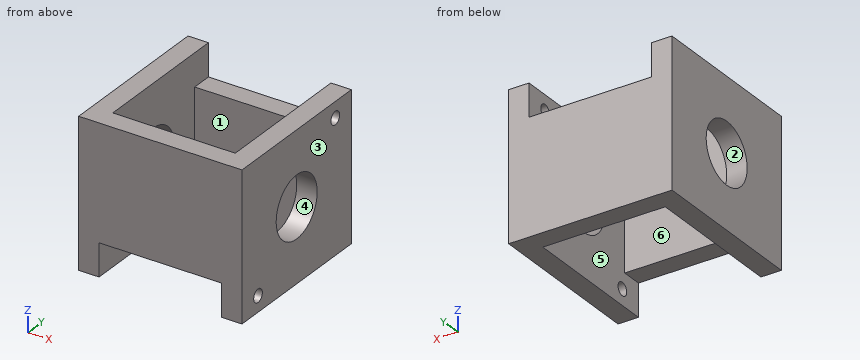
```python
from build123d import *

# Parameters (mm, degrees)
SKETCH1_W                      = 50.8
SKETCH1_H                      = 50.8
SKETCH1_W_2                    = 38.1
SKETCH1_H_2                    = 38.1
EXTRUDE_THIN1_DEPTH            = 45.72
SKETCH2_R                      = 2.0193
CUT_EXTRUDE2_DEPTH             = 1
CUT_EXTRUDE2_DEPTH_BACK        = 6.35
SKETCH4_R                      = 9.525
CUT_EXTRUDE3_DEPTH             = 1
CUT_EXTRUDE3_DEPTH_BACK        = 51.8
CUT_EXTRUDE4_REACH             = 52.8
SKETCH5_W                      = 38.1
SKETCH5_H                      = 10.16
CUT_EXTRUDE4_DIRECTION_2_DEPTH = 1
CUT_EXTRUDE5_START             = -25.4
SKETCH5_3_W                    = 38.1
SKETCH5_3_H                    = 10.16
CUT_EXTRUDE5_DEPTH             = 25.4


with BuildPart() as part:
    # Sketch1 → Extrude-Thin1 (new body)
    with BuildSketch(Plane.XY):
        Rectangle(SKETCH1_W, SKETCH1_H)
        Rectangle(SKETCH1_W_2, SKETCH1_H_2, mode=Mode.SUBTRACT)
    extrude(amount=EXTRUDE_THIN1_DEPTH)

    # Sketch2 → Cut-Extrude2 (cut, two sides)
    with BuildSketch(Plane(origin=(25.4, 0, 0), x_dir=(0, 0, -1), z_dir=(1, 0, 0))) as cut_extrude2_sk:
        with Locations((-40.820512212, 17.96051224)):
            Circle(SKETCH2_R)
        with Locations((-4.899487788, -17.96051224)):
            Circle(SKETCH2_R)
    extrude(amount=CUT_EXTRUDE2_DEPTH, mode=Mode.SUBTRACT)
    extrude(cut_extrude2_sk.sketch, amount=-CUT_EXTRUDE2_DEPTH_BACK, mode=Mode.SUBTRACT)

    # Sketch4 → Cut-Extrude3 (cut, two sides)
    with BuildSketch(Plane(origin=(25.4, 0, 0), x_dir=(0, 0, -1), z_dir=(1, 0, 0))) as cut_extrude3_sk:
        with Locations((-22.86, 0)):
            Circle(SKETCH4_R)
    extrude(amount=CUT_EXTRUDE3_DEPTH, mode=Mode.SUBTRACT)
    extrude(cut_extrude3_sk.sketch, amount=-CUT_EXTRUDE3_DEPTH_BACK, mode=Mode.SUBTRACT)

    # Sketch5 → Cut-Extrude4 (cut, up to next)
    with BuildSketch(Plane.XZ.offset(25.4), mode=Mode.PRIVATE) as cut_extrude4_sk1:
        with Locations((0, 5.08)):
            Rectangle(SKETCH5_W, SKETCH5_H)
    cut_extrude4_tool1 = extrude(cut_extrude4_sk1.sketch, amount=-CUT_EXTRUDE4_REACH, mode=Mode.PRIVATE) & part.part
    add(cut_extrude4_tool1.solids().sort_by_distance((0, -25.4, 5.08))[0], mode=Mode.SUBTRACT)

    # Sketch5 → Cut-Extrude4 direction 2 (cut)
    with BuildSketch(Plane.XZ.offset(25.4)):
        with Locations((0, 5.08)):
            Rectangle(SKETCH5_W, SKETCH5_H)
    extrude(amount=CUT_EXTRUDE4_DIRECTION_2_DEPTH, mode=Mode.SUBTRACT)

    # Sketch5<3> → Cut-Extrude5 (cut)
    with BuildSketch(Plane.XZ.offset(25.4).offset(CUT_EXTRUDE5_START)):
        with Locations((0, 40.64)):
            Rectangle(SKETCH5_3_W, SKETCH5_3_H)
    extrude(amount=-CUT_EXTRUDE5_DEPTH, mode=Mode.SUBTRACT)


solid = part.part
```
Geometry check sheet. Reference: the model listing, model coordinates, mm. Face numbers are marked on the shaded views. A direction names the side the tool comes from. Round coordinates to 2 decimals unless told otherwise and drop trailing zeros. Write each loop counter-clockwise with the first axis right and the second up, starting at its lowest first coordinate (ties: lowest second). Pieces come first, ordered by that corner, then holes. Notation, with made-up numbers: (66, 52.25) -> (115, 52.25) arc R8 ccw to (115, 60.25) -> close; hole circle Ø4 at (26.25, 5). An arc over 180 degrees is marked (long way). Put each result on its own line as item: value.
1) Cross-section at A-A, the plane y = 13. Enter the section's corners in (x, z).
Recorded:
outline: (-25.4, 0) -> (-19.05, 0) -> (-19.05, 45.72) -> (-25.4, 45.72) -> close; (19.05, 0) -> (25.4, 0) -> (25.4, 45.72) -> (19.05, 45.72) -> close
2) Cross-section at B-B, the plane y = 0. Enter the section's corners in (x, z) (3 decimals), plus the area to 3 significant figures.
Recorded:
outline: (-25.4, 0) -> (-19.05, 0) -> (-19.05, 13.335) -> (-25.4, 13.335) -> close; (-25.4, 32.385) -> (-19.05, 32.385) -> (-19.05, 45.72) -> (-25.4, 45.72) -> close; (19.05, 0) -> (25.4, 0) -> (25.4, 13.335) -> (19.05, 13.335) -> close; (19.05, 32.385) -> (25.4, 32.385) -> (25.4, 45.72) -> (19.05, 45.72) -> close
area: 339 mm2
3) Depth check by flat-ended pin: P1, Ø4, axis at x = 3.5, z = 6, coming from the -Y side; P2, Ø7, axis at x = 7, y = 23, coming from the +Z side; P3, Ø3, axis at x = 3, y = -23, coming from the -Z side. Enter the tip coordinate at first touch or a pass-through.
Recorded:
P1: stops at y = 19.05
P2: stops at z = 35.56
P3: stops at z = 10.16
4) Cross-section at C-C, the plane z = 22.86. Enter the section's corners in (x, y) (3 decimals).
Recorded:
outline: (-25.4, -25.4) -> (25.4, -25.4) -> (25.4, -9.525) -> (19.05, -9.525) -> (19.05, -19.05) -> (-19.05, -19.05) -> (-19.05, -9.525) -> (-25.4, -9.525) -> close; (-25.4, 9.525) -> (-19.05, 9.525) -> (-19.05, 19.05) -> (19.05, 19.05) -> (19.05, 9.525) -> (25.4, 9.525) -> (25.4, 25.4) -> (-25.4, 25.4) -> close
5) Release check for a two-part mould opening along X. For the marked faces 3, 4, 5 and 6 record: pulls with the +X half, pulls with the -X half, needs draft (parallel to the pull), parting line crosses it, or undercut.
Recorded:
face 3: pulls with the +X half
face 4: needs draft
face 5: undercut
face 6: undercut
6) Cross-section at D-D, the plane x = -11.5. Enter the section's corners in (y, z), plus the area to 3 significant figures.
Recorded:
outline: (-25.4, 10.16) -> (-19.05, 10.16) -> (-19.05, 45.72) -> (-25.4, 45.72) -> close; (19.05, 0) -> (25.4, 0) -> (25.4, 35.56) -> (19.05, 35.56) -> close
area: 452 mm2
7) Thickness scan on probe 1 along Y at (x, z) = (4, 13.5); probe 2 along Y at (x, z) = (22.5, 22.86) (3 decimals). Record the ranges inside material, lowest first. Write a range as from..to.
Recorded:
probe 1: y = -25.4..-19.05, 19.05..25.4
probe 2: y = -25.4..-9.525, 9.525..25.4
8) Access from +Z, -Z, +X, -X, +Y, -Y to the whole of each face (thin tool, end or side, straight path). Record for the marked faces 1 and 2.
Recorded:
face 1: +Z, -Z
face 2: +X, -X
